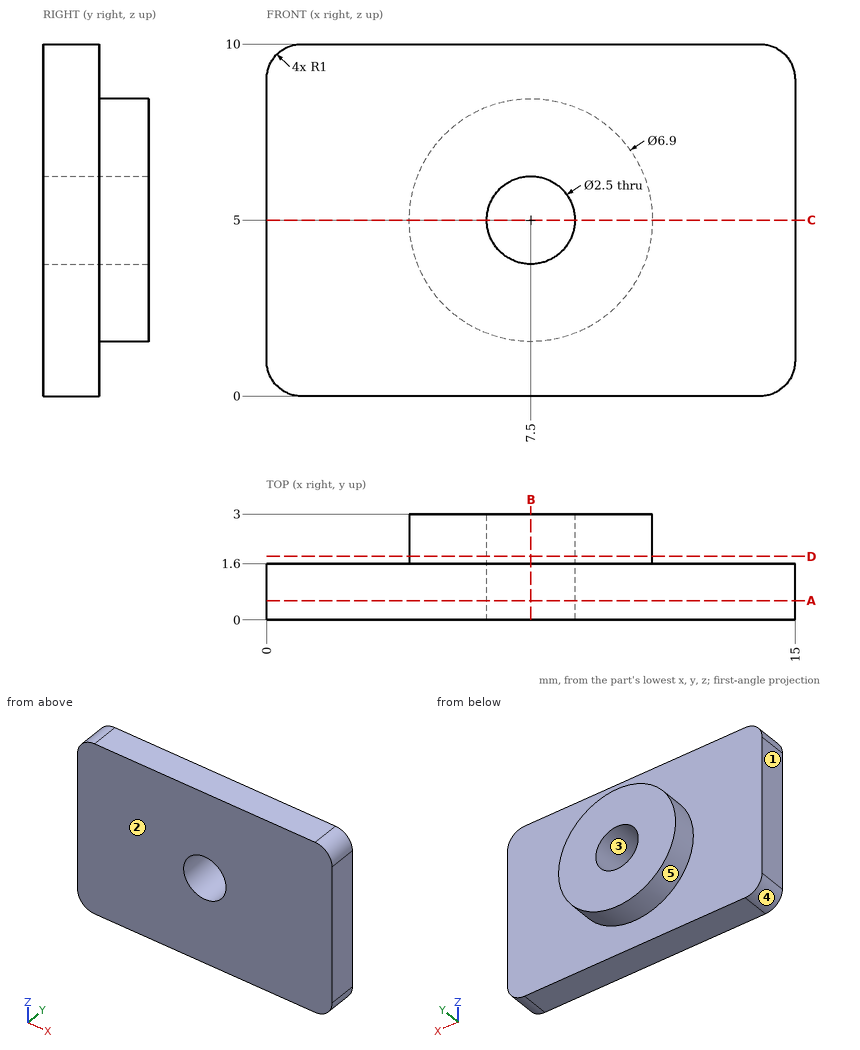
For this review, use the dimensioned drawing (mm, ordinates from the lowest corner) and the shaded views. A direction names the side the tool comes from. Coordinates: 2 decimals unless noted, no trailing zeros. Order: outer loops, then holes, each group sorted by start corner. A loop starts at its lowest first (then second) coordinate and runs counter-clockwise, first axis right, second up. Notation, with made-up numbers: (-3, -24.5) -> (23, -24.5) arc R25 ccw to (23, -0.5) -> close; hole circle Ø6 at (83.5, -26). An arc over 180 degrees is marked (long way). One line per item, written item: value. Start each with the question number.
Q1. Mouldability with a two-part tool opening along X and no side actions: class the marked faces 1, 2 and 3 as pulls with the +X half, pulls with the -X half, needs draft (parallel to the pull), parting line crosses it, or undercut.
Q2. Tool access review of the marked faces 4 and 5: name each direction out of +Z, -Z, +X, -X, +Y, -Y from which nothing blocks a thin tool from reaching the whole face with its end or side.
Q3. Take a section at D-D, the plane y = 1.8. State the section outline as (x, z) points.
Q4. Take a section at B-B, the plane x = 7.5. State the section outline as (y, z) points, then the cut area to 3 significant figures.
Q5. Insertion check: pin 1 Ø3 at (x, z) = (7.5, 5) entering from -Y. The pin has a flat end and moves straight along its axis. Give the tip position at first contact, or say it passes through.
Q6. Take a section at A-A, the plane y = 0.55. State the section outline as (x, z) points.
Q7. Take a section at C-C, the plane z = 5. State the section outline as (x, y) points.
Q8. For probe 1 along Z at (x, y) = (7.5, 0.9); probe 2 along X at (y, z) = (2.25, 5); probe 3 along X at (y, z) = (0.8, 5), list the stretches that pass through material, from the lowest coordinate up.
Values follow:
1. face 1: pulls with the -X half
1. face 2: needs draft
1. face 3: undercut
2. face 4: -Z, -X, +Y, -Y
2. face 5: +Y
3. outline: circle Ø6.9 at (7.5, 5); hole circle Ø2.5 at (7.5, 5)
4. outline: (0, 0) -> (1.6, 0) -> (1.6, 1.55) -> (3, 1.55) -> (3, 3.75) -> (0, 3.75) -> close; (0, 6.25) -> (3, 6.25) -> (3, 8.45) -> (1.6, 8.45) -> (1.6, 10) -> (0, 10) -> close
4. area: 18.2 mm2
5. pin 1: stops at y = 0
6. outline: (0, 1) arc R1 ccw to (1, 0) -> (14, 0) arc R1 ccw to (15, 1) -> (15, 9) arc R1 ccw to (14, 10) -> (1, 10) arc R1 ccw to (0, 9) -> close; hole circle Ø2.5 at (7.5, 5)
7. outline: (0, 0) -> (6.25, 0) -> (6.25, 3) -> (4.05, 3) -> (4.05, 1.6) -> (0, 1.6) -> close; (8.75, 0) -> (15, 0) -> (15, 1.6) -> (10.95, 1.6) -> (10.95, 3) -> (8.75, 3) -> close
8. probe 1: z = 0 to 3.75, 6.25 to 10
8. probe 2: x = 4.05 to 6.25, 8.75 to 10.95
8. probe 3: x = 0 to 6.25, 8.75 to 15
